Check sheet for the modelled part. Datum: model origin and axes. Units: mm. Face numbers are marked on the shaded views. Round coordinates to 2 decimals unless told otherwise and drop trailing zeros. Order: outer loops, then holes, each group sorted by start corner. A loop starts at its lowest first (then second) coordinate and runs counter-clockwise, first axis right, second up. Notation, with made-up numbers: (-35, -1.75) -> (-14, -1.75) arc R22 ccw to (-14, 27.25) -> close; hole circle Ø10 at (-16.75, 68.5). An arc over 180 degrees is marked (long way). Answer in a Markdown table with one row per item.
from build123d import *

# Parameters (mm, degrees)
RESSALTO_EXTRUS_O1_DEPTH = 57
CORTE_EXTRUS_O1_START    = -11
CORTE_EXTRUS_O1_DEPTH    = 11
CORTE_EXTRUS_O2_DEPTH    = 11


with BuildPart() as part:
    # Esboço1 → Ressalto-extrusão1 (new body)
    with BuildSketch(Plane(origin=(0, 0, 0), x_dir=(1, 0, 0), z_dir=(0, 1, 0))):
        with BuildLine():
            Line((-47, 0), (47, 0))
            ThreePointArc((47, 0), (47.85009345, 3.078711179), (50.159487509, 5.285024956))
            ThreePointArc((50.159487509, 5.285024956), (52.004661638, 4.729916917), (51.449553599, 2.884742789))
            ThreePointArc((51.449553599, 2.884742789), (52.536782743, -3.242075689), (55.296246294, 2.335139815))
            ThreePointArc((55.296246294, 2.335139815), (56.096189798, 3.978813584), (57.863892701, 3.513196237))
            ThreePointArc((57.863892701, 3.513196237), (58.342245662, -2.731375348), (53, -6))
            Line((53, -6), (-53, -6))
            ThreePointArc((-53, -6), (-58.342245662, -2.731375348), (-57.863892701, 3.513196237))
            ThreePointArc((-57.863892701, 3.513196237), (-56.096189798, 3.978813584), (-55.296246294, 2.335139815))
            ThreePointArc((-55.296246294, 2.335139815), (-52.536782743, -3.242075689), (-51.449553599, 2.884742789))
            ThreePointArc((-51.449553599, 2.884742789), (-52.004661638, 4.729916917), (-50.159487509, 5.285024956))
            ThreePointArc((-50.159487509, 5.285024956), (-47.85009345, 3.078711179), (-47, 0))
        make_face()
    extrude(amount=RESSALTO_EXTRUS_O1_DEPTH)

    # Esboço2 → Corte-extrusão1 (cut)
    with BuildSketch(Plane(origin=(0, 57, 0), x_dir=(1, 0, 0), z_dir=(0, 1, 0)).offset(CORTE_EXTRUS_O1_START)):
        with BuildLine():
            Line((47, 0), (47, -6))
            Line((47, -6), (53, -6))
            ThreePointArc((53, -6), (57.242640687, 4.242640687), (47, 0))
        make_face()
        with BuildLine():
            Line((-47, 0), (-47, -6))
            Line((-47, -6), (-53, -6))
            ThreePointArc((-53, -6), (-57.242640687, 4.242640687), (-47, 0))
        make_face()
    extrude(amount=CORTE_EXTRUS_O1_DEPTH, mode=Mode.SUBTRACT)

    # Esboço3 → Corte-extrusão2 (cut)
    with BuildSketch(Plane.XZ):
        with BuildLine():
            Line((-47, 0), (-47, 6))
            Line((-47, 6), (-53, 6))
            ThreePointArc((-53, 6), (-57.242640687, -4.242640687), (-47, 0))
        make_face()
        with BuildLine():
            Line((47, 0), (47, 6))
            Line((47, 6), (53, 6))
            ThreePointArc((53, 6), (57.242640687, -4.242640687), (47, 0))
        make_face()
    extrude(amount=-CORTE_EXTRUS_O2_DEPTH, mode=Mode.SUBTRACT)


solid = part.part
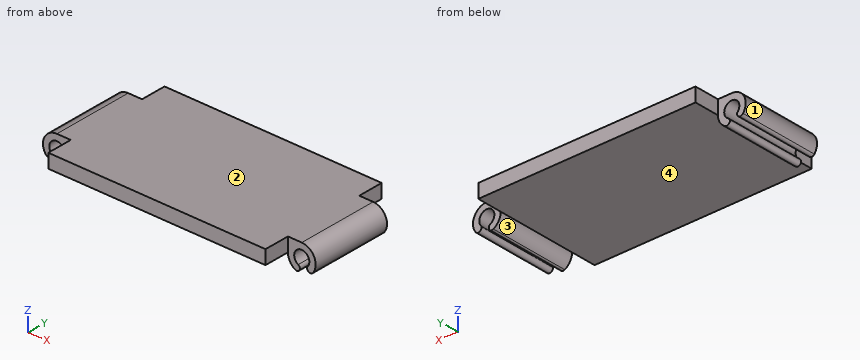
Item 1: Scan lines: line 1 (X direction, y = 40.5, z = 3); line 2 (Z direction, x = -13.5, y = 46.5); line 3 (Z direction, x = 53, y = 36.5) (3 decimals). Record each from-to range of solid material in increasing order. Write a range as [from, to].
Result sheet:
| item | result |
|---|---|
| line 1 | x = [-58.2, -54.31], [-51.69, 51.69], [54.31, 58.2] |
| line 2 | z = [0, 6] |
| line 3 | z = [3.275, 6] |
Item 2: Mould release check, pull along X, two halves, no side actions. Record for the marked faces 1, 2, 3 and 4: pulls with the +X half, pulls with the -X half, needs draft (parallel to the pull), parting line crosses it, or undercut.
Result sheet:
| item | result |
|---|---|
| face 1 | pulls with the -X half |
| face 2 | needs draft |
| face 3 | undercut |
| face 4 | undercut |
Item 3: Depth check by flat-ended pin: P1, Ø3, axis at y = 5, z = 4, coming from the -X side; P2, Ø2, axis at y = 41, z = 4.5, coming from the -X side; P3, Ø17, axis at x = 16.5, y = 17, coming from the -Z side. Enter the tip coordinate at first touch or a pass-through.
Result sheet:
| item | result |
|---|---|
| P1 | stops at x = -47 |
| P2 | stops at x = -57.87 |
| P3 | stops at z = 0 |
Item 4: Cross-section at A-A (y = 52.5). Record the boundary of the cut face in (x, z).
Result sheet:
| item | result |
|---|---|
| outline | (-47, 0) -> (47, 0) -> (47, 6) -> (-47, 6) -> close |
Item 5: Cross-section at B-B (x = -40). Record the boundary of the cut face in (y, z).
Result sheet:
| item | result |
|---|---|
| outline | (0, 0) -> (57, 0) -> (57, 6) -> (0, 6) -> close |
